from build123d import *

# Parameters (mm, degrees)
F2_R     = 2
F4_DEPTH = 3
F5_DEPTH = 5


with BuildPart() as f1:
    # F0 (on Top) → F1 (revolve)
    with BuildSketch(Plane.XY):
        Polygon((0.6408938694, 3), (0.6408938694, 16.7043862722), (-11.46528483, 16.7043862722), (-13.8516243371, 0), (-12.3516243371, 0), (-10.3318675491, 14.1383057447), (-3.8579331173, 14.1383057447), (-3.8579331173, 3), align=None)
    revolve(axis=Axis((0.6408938694, 3.1900271702, 0), (0, -1, 0)))

    # F2
    f2_edges = [f1.edges().sort_by_distance(p)[0] for p in [
        (12.747073, 16.704386, 0),
    ]]
    fillet(f2_edges, radius=F2_R)

    # F3 (on face) → F4 (cut)
    with BuildSketch(Plane.XZ.offset(-3)):
        with BuildLine():
            ThreePointArc((2.2408938694, -2.6551836095), (3.3399677847, -1.5247950682), (3.7408938694, 0))
            ThreePointArc((3.7408938694, 0), (3.3399677847, 1.5247950682), (2.2408938694, 2.6551836095))
            Line((2.2408938694, 2.6551836095), (2.2408938694, -2.6551836095))
        make_face()
        with BuildLine():
            Line((2.2408938694, -2.6551836095), (2.2408938694, 2.6551836095))
            ThreePointArc((2.2408938694, 2.6551836095), (-2.4591061306, 0), (2.2408938694, -2.6551836095))
        make_face()
    extrude(amount=-F4_DEPTH, mode=Mode.SUBTRACT)

    # F3 (on face) → F5 (cut)
    with BuildSketch(Plane.XZ.offset(-3)):
        with BuildLine():
            Line((2.2408938694, -2.6551836095), (2.2408938694, 2.6551836095))
            ThreePointArc((2.2408938694, 2.6551836095), (-2.4591061306, 0), (2.2408938694, -2.6551836095))
        make_face()
    extrude(amount=-F5_DEPTH, mode=Mode.SUBTRACT)


solid = f1.part
Could you check a few things on this model? Use its own coordinates, in mm. A direction names the side the tool comes from. Round coordinates to 2 decimals unless told otherwise and drop trailing zeros. Loops run counter-clockwise (first coordinate to the right, second up) from the corner with the lowest first, then second, coordinate; pieces in that order, holes last. Notation, with made-up numbers: (-19.5, 34.25) - (37.5, 34.25) arc R23 cw to (37.5, 69.25) - close; hole circle Ø7 at (38.25, 24). An arc over 180 degrees is marked (long way). Write item = value, one per line.
1) If we mould it in two halves opening along Z, with no side actions, what happens to faces 3 (the flat face through (-4.1, 14.138, -0.2)), 4 (the conical face through (11.115, 9.054, 8.031)), 5 (the flat face through (0, 16.704, 0))? For each: pulls with the +Z half, pulls with the -Z half, needs draft (parallel to the pull), parting line crosses it, or undercut.
Computed:
face_3 = undercut
face_4 = parting line crosses it
face_5 = needs draft
2) On a 3-axis mill with a long thin cutter (end or side, diameter ignored), from which of +Z, -Z, +X, -X, +Y, -Y can I reach the whole of each face in a straight line? I mean faces 1 (the flat face through (3, 0, -13)), 2 (the flat face through (2, 3, 3)). Say none if no direction works.
Computed:
face_1 = +Z, -Z, +X, -X, -Y
face_2 = -Y
3) Imagine slicing it at B-B (y = 12.5). Please give me the cut outline in (x, z), and give its area (3 significant figures).
Computed:
outline = circle Ø25.41 at (0.64, 0); circle Ø9 at (0.64, 0); hole circle Ø22.41 at (0.64, 0)
area = 176 mm2
4) I'm going to push flat-ended pins straight in: P1, Ø5, axis at x = -5.5, y = 7, coming from the -Z side; P2, Ø5, axis at x = 2, y = 12.5, coming from the -Z side; P3, Ø5, axis at x = 10.5, y = 7, coming from the -Z side. Where does each tip first touch, or does it pass through?
Computed:
P1 = -13.08
P2 = -13.03
P3 = -11.36
5) I need wall thicknesses on line 1 along X through (y, z) = (5.8, 0); line 2 along X through (y, z) = (14, 3.5); line 3 along X through (y, z) = (6.35, 0). Which ranges of each line are inside material? Lowest first, please. Write a range as from..to.
Computed:
line_1 = -13.02..-11.52, -3.86..-2.46, 3.74..5.14, 12.8..14.3
line_2 = -11.35..-9.78, -2.19..3.47, 11.06..12.63
line_3 = -12.94..-11.44, -3.86..-2.46, 2.24..5.14, 12.73..14.23
6) Imagine slicing it at D-D (y = 9.5). Please give me the cut outline in (x, z), and give its area (3 significant figures).
Computed:
outline = circle Ø26.27 at (0.64, 0); circle Ø9 at (0.64, 0); hole circle Ø23.27 at (0.64, 0)
area = 180 mm2
7) Imagine slicing it at A-A (y = 3.5). Please give me the cut outline in (x, z), and give its area (3 significant figures).
Computed:
outline = circle Ø27.99 at (0.64, 0); circle Ø9 at (0.64, 0); hole circle Ø24.99 at (0.64, 0); hole circle Ø6.2 at (0.64, 0)
area = 158 mm2
8) Imagine slicing it at C-C (y = 5.25). Please give me the cut outline in (x, z), and give its area (3 significant figures).
Computed:
outline = circle Ø27.49 at (0.64, 0); circle Ø9 at (0.64, 0); hole circle Ø24.49 at (0.64, 0); hole circle Ø6.2 at (0.64, 0)
area = 156 mm2
